Here's how the part is built. I have some questions about the finished solid (model axes, mm). Face numbers are marked on the shaded views. A direction names the side the tool comes from. Give positions to 0.01 mm unless a question says otherwise; leave off trailing zeros. Loops run counter-clockwise (first coordinate to the right, second up) from the corner with the lowest first, then second, coordinate; pieces in that order, holes last. Notation, with made-up numbers: (-39, 15) - (2, 15) arc R22 ccw to (2, 54) - close; hole circle Ø5 at (53.5, 69.5). An arc over 180 degrees is marked (long way). Use a Markdown table: item, result.
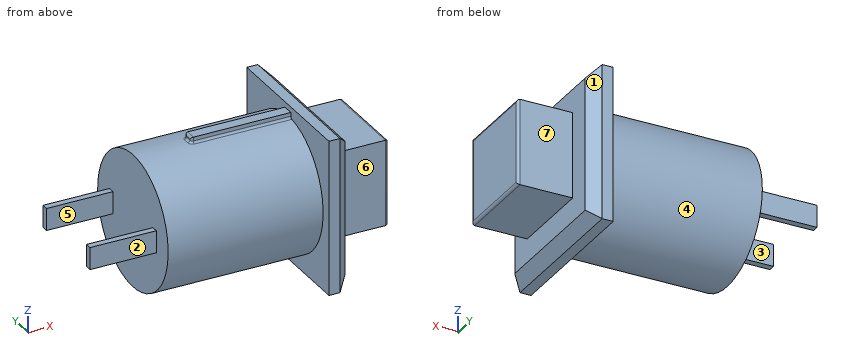
from build123d import *

# Parameters (mm, degrees)
F0_R      = 6
F1_DEPTH  = 14
F2_W      = 14
F2_H      = 14
F3_DEPTH  = 2
F4_W      = 7.75
F4_H      = 7.75
F5_DEPTH  = 5
F6_W      = 0.6
F6_H      = 2
F7_DEPTH  = 6
F8_R      = 0.25
F9_SIZE   = 1
F11_DEPTH = 9
F12_R     = 0.2


with BuildPart() as f1:
    # F0 (on Right) → F1 (new body)
    with BuildSketch(Plane.YZ):
        Circle(F0_R)
    extrude(amount=F1_DEPTH)

    # F2 (on face) → F3 (join)
    with BuildSketch(Plane.YZ.offset(14)):
        Rectangle(F2_W, F2_H)
    extrude(amount=F3_DEPTH)

    # F4 (on face) → F5 (join)
    with BuildSketch(Plane.YZ.offset(16)):
        Rectangle(F4_W, F4_H)
    extrude(amount=F5_DEPTH)

    # F6 (on face) → F7 (join)
    with BuildSketch(Plane(origin=(0, 0, 0), x_dir=(0, -1, 0), z_dir=(-1, 0, 0))):
        with Locations((-3.7, 0)):
            Rectangle(F6_W, F6_H)
        with Locations((3.7, 0)):
            Rectangle(F6_W, F6_H)
    extrude(amount=F7_DEPTH)

    # F8
    f8_edges = [f1.edges().sort_by_distance(p)[0] for p in [
        (21, 0, 3.875),
        (21, -3.875, 0),
        (21, 0, -3.875),
        (21, 3.875, 0),
    ]]
    fillet(f8_edges, radius=F8_R)

    # F9
    f9_edges = [f1.edges().sort_by_distance(p)[0] for p in [
        (16, 0, -7),
        (16, -7, 0),
        (16, 0, 7),
        (16, 7, 0),
    ]]
    chamfer(f9_edges, length=F9_SIZE)

    # F10 (on face) → F11 (join)
    with BuildSketch(Plane(origin=(14, 0, 0), x_dir=(0, -1, 0), z_dir=(-1, 0, 0))):
        Polygon((0.5, 6.5), (-0.5, 6.5), (-0.5, 6), (-0.5, 5.9002675116), (0.5, 5.9002675116), (0.5, 6), align=None)
    extrude(amount=F11_DEPTH)

    # F12
    f12_edges = [f1.edges().sort_by_distance(p)[0] for p in [
        (5, -0.5, 6.239565),
        (5, 0, 6),
        (5, 0.5, 6.239565),
        (5, 0, 6.5),
        (9.5, -0.5, 5.97913),
        (9.5, 0.5, 5.97913),
    ]]
    fillet(f12_edges, radius=F12_R)


solid = f1.part
(1) If I drill on line 1 (X direction, y = -1.25, z = -4.5); line 2 (X direction, y = 1, z = -2.75); line 3 (Y direction, x = 16.25, z = 3.5) (3 decimals), over which ranges is the centre line in solid material (lowest first)?
A:
| item | result |
|---|---|
| line 1 | 0 to 16 |
| line 2 | 0 to 21 |
| line 3 | -3.875 to 3.875 |
(2) Suppose I cut it at B-B on y = 0. Write out the boundary of the cut face in (x, z) (3 decimals), plus the area to 3 significant figures.
A:
| item | result |
|---|---|
| outline | (0, -6) - (14, -6) - (14, -7) - (15, -7) - (16, -6) - (16, -3.875) - (20.75, -3.875) arc R0.25 ccw to (21, -3.625) - (21, 3.625) arc R0.25 ccw to (20.75, 3.875) - (16, 3.875) - (16, 6) - (15, 7) - (14, 7) - (14, 6.5) - (5.2, 6.5) arc R0.2 ccw to (5, 6.3) - (5, 6.2) arc R0.2 cw to (4.8, 6) - (0, 6) - close |
| area | 238 mm2 |
(3) Suppose I cut it at D-D on x = 1. Write out the boundary of the cut face in (y, z), plus the area to 3 significant figures.
A:
| item | result |
|---|---|
| outline | circle Ø12 at (0, 0) |
| area | 113 mm2 |
(4) Will these pins go through, and if not, where does the flat tip stop? pin 1 (4 mm diameter, centred on x = 10.5, y = -4.5, fed in from +Z); pin 2 (5 mm diameter, centred on y = -5, z = -1.5, fed in from -X); pin 3 (1.5 mm diameter, centred on y = 2.5, z = -0.5, fed in from -X); pin 4 (1.4 mm diameter, centred on x = 19, y = -2, fed in from -Z) (3 decimals).
A:
| item | result |
|---|---|
| pin 1 | z = 5.45 |
| pin 2 | x = -6 |
| pin 3 | x = 0 |
| pin 4 | z = -3.875 |
(5) Suppose I cut it at A-A on z = 0. Write out the boundary of the cut face in (x, y) (3 decimals).
A:
| item | result |
|---|---|
| outline | (-6, -4) - (0, -4) - (0, -6) - (14, -6) - (14, -7) - (15, -7) - (16, -6) - (16, -3.875) - (20.75, -3.875) arc R0.25 ccw to (21, -3.625) - (21, 3.625) arc R0.25 ccw to (20.75, 3.875) - (16, 3.875) - (16, 6) - (15, 7) - (14, 7) - (14, 6) - (0, 6) - (0, 4) - (-6, 4) - (-6, 3.4) - (0, 3.4) - (0, -3.4) - (-6, -3.4) - close |
(6) On a 3-axis mill with a long thin cutter (end or side, diameter ignored), from which of +Z, -Z, +X, -X, +Y, -Y can I reach the whole of each face in a straight line? I mean the marked faces 4, 5, 6 and 7. Say none if no direction works.
A:
| item | result |
|---|---|
| face 4 | -X |
| face 5 | +Z, -Z, -X |
| face 6 | +Z, -Z, +X, -Y |
| face 7 | +Z, -Z, +X, +Y |
(7) Suppose I cut it at C-C on x = 8.5. Write out the boundary of the cut face in (y, z), plus the area to 3 significant figures.
A:
| item | result |
|---|---|
| outline | (-0.68, 5.96) arc R6 ccw (long way) to (0.68, 5.96) arc R0.2 cw to (0.5, 6.16) - (0.5, 6.5) - (-0.5, 6.5) - (-0.5, 6.16) arc R0.2 cw to start |
| area | 114 mm2 |
(8) We'd pull the mould along Y, two halves only. Please class the marked faces 1, 2 and 3: pulls with the +Y half, pulls with the -Y half, needs draft (parallel to the pull), parting line crosses it, or undercut.
A:
| item | result |
|---|---|
| face 1 | pulls with the +Y half |
| face 2 | pulls with the -Y half |
| face 3 | undercut |
